```python
from build123d import *

# Parameters (mm, degrees)
F1_DEPTH  = 7
F3_R      = 18.475
F4_DEPTH  = 25
F5_W      = 25
F5_H      = 7
F6_DEPTH  = 30
F7_W      = 25
F7_H      = 7
F8_DEPTH  = 30
F9_W      = 25
F9_H      = 7
F10_DEPTH = 30
F12_DEPTH = 25
F14_DEPTH = 25
F16_DEPTH = 25
F17_R     = 5


with BuildPart() as f1:
    # F0 (on Top) → F1 (new body)
    with BuildSketch(Plane.XY):
        Polygon((-20, 34.6410161514), (0, 23.0940107676), (0, 69.2820323028), align=None)
        Polygon((0, 23.0940107676), (20, 34.6410161514), (0, 69.2820323028), align=None)
        Polygon((0, 23.0940107676), (40, 0), (20, 34.6410161514), align=None)
        Polygon((0, 0), (40, 0), (0, 23.0940107676), align=None)
        Polygon((-40, 0), (0, 0), (0, 23.0940107676), align=None)
        Polygon((-40, 0), (0, 23.0940107676), (-20, 34.6410161514), align=None)
    extrude(amount=F1_DEPTH)


with BuildPart() as f1_1:
    # F2: moved
    add(f1.part.moved(Location((0, -23.09401, 0))))

    # F3 (on face) → F4 (cut)
    with BuildSketch(Plane.XY.offset(7)):
        Circle(F3_R)
    extrude(amount=-F4_DEPTH, mode=Mode.SUBTRACT)

    # F5 (on face) → F6 (join)
    with BuildSketch(Plane.XZ.offset(23.09401)):
        with Locations((0, 3.5)):
            Rectangle(F5_W, F5_H)
    extrude(amount=F6_DEPTH)

    # F7 (on face) → F8 (join)
    with BuildSketch(Plane(origin=(20.0000003324, 11.5470055757, 0), x_dir=(-0.5, 0.8660254038, 0), z_dir=(0.8660254038, 0.5, 0))):
        with Locations((6.647e-07, 3.5)):
            Rectangle(F7_W, F7_H)
    extrude(amount=F8_DEPTH)

    # F9 (on face) → F10 (join)
    with BuildSketch(Plane(origin=(-20.0000003324, 11.5470055757, 0), x_dir=(-0.5, -0.8660254038, 0), z_dir=(-0.8660254038, 0.5, 0))):
        with Locations((0, 3.5)):
            Rectangle(F9_W, F9_H)
    extrude(amount=F10_DEPTH)

    # F11 (on face) → F12 (cut)
    with BuildSketch(Plane.XY.offset(7)):
        Polygon((0, 46.1880223028), (-13.7500003324, 22.372323123), (13.75, 22.3723236987), align=None)
        Polygon((26.25, 0.7216886041), (12.5, -23.09401), (40, -23.09401), align=None)
        Polygon((-12.5, -23.09401), (-26.2500003324, 0.7216880284), (-40, -23.09401), align=None)
    extrude(amount=-F12_DEPTH, mode=Mode.SUBTRACT)

    # F13 (on face) → F14 (cut)
    with BuildSketch(Plane.XY.offset(7)):
        with BuildLine():
            ThreePointArc((-22.8564067929, 19.5470055757), (-31.0093972968, 30.1721896649), (-43.3826862346, 25.0470055757))
            ThreePointArc((-43.3826862346, 25.0470055757), (-36.7034162891, 8.9218214865), (-22.8564067929, 19.5470055757))
        make_face()
        with BuildLine():
            ThreePointArc((44.8564064606, 19.5470061514), (44.4815905497, 22.3940156475), (43.3826859022, 25.0470061514))
            ThreePointArc((43.3826859022, 25.0470061514), (23.2312223714, 16.6999966552), (44.8564064606, 19.5470061514))
        make_face()
        with BuildLine():
            ThreePointArc((11, -39.09401), (-7.7781745931, -31.3158354069), (0, -50.09401))
            ThreePointArc((0, -50.09401), (7.7781745931, -46.8721845931), (11, -39.09401))
        make_face()
    extrude(amount=-F14_DEPTH, mode=Mode.SUBTRACT)

    # F15 (on face) → F16 (cut)
    with BuildSketch(Plane.XY.offset(7)):
        Polygon((-20.2451908608, 26.122323123), (-16.8750003324, 16.9596643493), (-13.7500003324, 22.372323123), align=None)
        Polygon((-13.7500003324, 22.372323123), (-16.8750003324, 16.9596643493), (-1.662e-07, 22.3723234108), align=None)
        Polygon((13.75, 22.3723236987), (-1.662e-07, 22.3723234108), (16.875, 16.959664925), align=None)
        Polygon((13.75, 22.3723236987), (16.875, 16.959664925), (20.2451905284, 26.1223236987), align=None)
        Polygon((32.7451905284, 4.4716886041), (23.125, 6.1343473777), (26.25, 0.7216886041), align=None)
        Polygon((23.125, 6.1343473777), (19.375, -11.186160698), (26.25, 0.7216886041), align=None)
        Polygon((19.375, -11.186160698), (6.25, -23.09401), (12.5, -23.09401), align=None)
        Polygon((12.5, -23.09401), (6.25, -23.09401), (12.5, -30.59401), align=None)
        Polygon((-12.5, -29.9828486929), (-6.25, -23.09401), (-12.5, -23.09401), align=None)
        Polygon((-6.25, -23.09401), (-19.3750001662, -11.1861609858), (-12.5, -23.09401), align=None)
        Polygon((-23.1250003324, 6.134346802), (-26.2500003324, 0.7216880284), (-19.3750001662, -11.1861609858), align=None)
        Polygon((-32.7451908608, 4.4716880284), (-26.2500003324, 0.7216880284), (-23.1250003324, 6.134346802), align=None)
        Polygon((-52.2307624459, 15.7216880284), (-45.7355719175, 11.9716880284), (-49.1057624459, 21.134346802), align=None)
        Polygon((-42.8557624459, 31.9596643493), (-33.2355719175, 33.622323123), (-39.7307624459, 37.372323123), align=None)
        Polygon((39.7307621135, 37.3723236987), (33.2355715851, 33.6223236987), (42.8557621135, 31.959664925), align=None)
        Polygon((49.1057621135, 21.1343473777), (45.7355715851, 11.9716886041), (52.2307621135, 15.7216886041), align=None)
        Polygon((12.5, -53.09401), (12.5, -45.59401), (6.25, -53.09401), align=None)
        Polygon((-6.25, -53.09401), (-12.5, -45.59401), (-12.5, -53.09401), align=None)
    extrude(amount=-F16_DEPTH, mode=Mode.SUBTRACT)

    # F17
    f17_edges = [f1_1.edges().sort_by_distance(p)[0] for p in [
        (6.25, -53.09401, 3.5),
        (12.5, -45.59401, 3.5),
        (12.5, -30.59401, 3.5),
        (-6.25, -53.09401, 3.5),
        (23.125, 6.134347, 3.5),
        (32.745191, 4.471689, 3.5),
        (45.735572, 11.971689, 3.5),
        (6.25, -23.09401, 3.5),
        (49.105762, 21.134347, 3.5),
        (42.855762, 31.959665, 3.5),
        (33.235572, 33.622324, 3.5),
        (20.245191, 26.122324, 3.5),
        (-33.235572, 33.622323, 3.5),
        (-12.5, -29.982849, 3.5),
        (-42.855762, 31.959664, 3.5),
        (-49.105762, 21.134347, 3.5),
        (-16.875, 16.959664, 3.5),
        (-23.125, 6.134347, 3.5),
        (-32.745191, 4.471688, 3.5),
        (-45.735572, 11.971688, 3.5),
        (-6.25, -23.09401, 3.5),
        (-19.375, -11.186161, 3.5),
        (0, 22.372323, 3.5),
        (16.875, 16.959665, 3.5),
        (19.375, -11.186161, 3.5),
    ]]
    fillet(f17_edges, radius=F17_R)


solid = f1_1.part
```
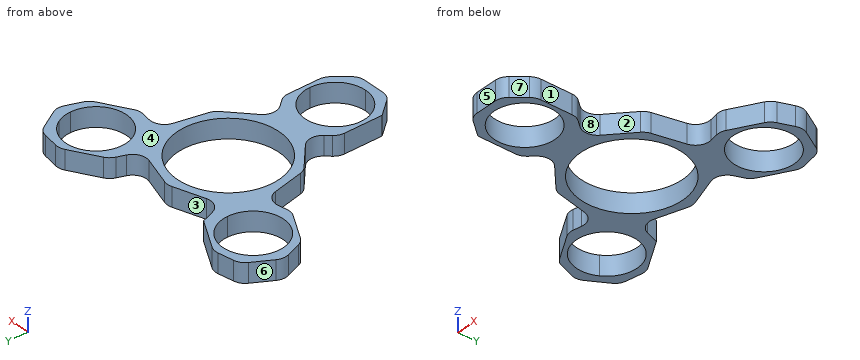
Input: part model. Units: mm. Frame: model coordinates. Face numbers are marked on the shaded views. A direction names the side the tool comes from. Round coordinates to 2 decimals unless told otherwise and drop trailing zeros. Loops run counter-clockwise (first coordinate to the right, second up) from the corner with the lowest first, then second, coordinate; pieces in that order, holes last. Notation, with made-up numbers: (49.25, 73) -> (77.25, 73) arc R24 ccw to (77.25, 102) -> close; hole circle Ø9 at (89.25, 56). An arc over 180 degrees is marked (long way). Use one line per item in the form item = value. Start each with the question number.
Item 1: Set-up query: the marked faces 1, 2, 3, 4 and 5. Return all of +Z, -Z, +X, -X, +Y, -Y with unobstructed straight access to the full face (end or side cutting, diameter ignored); none if empty.
Item 2: Section query B-B on y = 0. Return the cut outline in (x, z) (3 decimals), then the cut area to 3 significant figures.
Item 3: Material intervals for L1, parallel to Y at x = 9, z = 5.75; L2, parallel to X at y = -39.5, z = 3.5; L3, parallel to Y at x = 12, z = 4.75, sorted ascending. Write a range as from..to.
Item 4: Contact query for flat-ended pins moving along their axis: pin 1 Ø1 at (x, z) = (-28, 1.5) entering from -Y; pin 2 Ø2 at (x, z) = (-15.5, 6) entering from -Y; pin 3 Ø2 at (y, z) = (-36, 5) entering from -X. Output: stop coordinate, or through.
Item 5: Section query C-C on z = 2.75. Count the separate pieces of the cut face and the enclosed holes in it, then the cut area to 3 significant figures.
Item 6: Section query A-A on x = -42. Return the cut outline in (y, z).
Item 7: Mould query, pull axis Y, two halves, no side actions, for the marked faces 6, 7 and 8. Classes: pulls with the +Y half, pulls with the -Y half, needs draft (parallel to the pull), parting line crosses it, or undercut.
Ans:
q1.face_1 = +Z, -Z, +X, -Y
q1.face_2 = +Z, -Z, +X
q1.face_3 = +Z, -Z, +Y
q1.face_4 = +Z, +X, -X, +Y, -Y
q1.face_5 = +Z, -Z, +X, -X, -Y
q2.outline = (-21.797, 0) -> (-18.475, 0) -> (-18.475, 7) -> (-21.797, 7) -> close; (18.475, 0) -> (21.797, 0) -> (21.797, 7) -> (18.475, 7) -> close
q2.area = 46.5 mm^2
q3.L1 = -49.79..-45.42, -32.77..-26.35, -20.8..-16.13, 16.13..19.49
q3.L2 = -12.5..-10.99, 10.99..12.5
q3.L3 = -45.96..-30.22, -17.88..-14.05, 14.05..18.52
q4.pin_1 = 5.21
q4.pin_2 = -15.61
q4.pin_3 = -12.5
q5.separate_pieces = 1
q5.enclosed_holes = 4
q5.area = 1,340 mm^2
q6.outline = (9.81, 0) -> (12.15, 0) -> (12.15, 7) -> (9.81, 7) -> close; (26.94, 0) -> (31.87, 0) -> (31.87, 7) -> (26.94, 7) -> close
q7.face_6 = pulls with the +Y half
q7.face_7 = pulls with the -Y half
q7.face_8 = undercut
